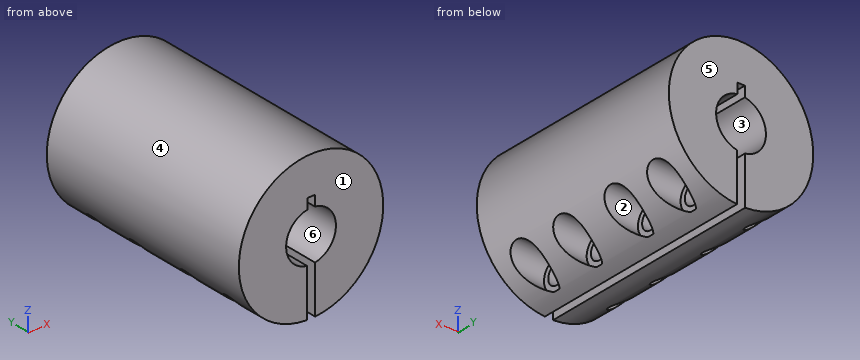
```python
from build123d import *

# Parameters (mm, degrees)
SKETCH1_R           = 14.5
SKETCH1_R_2         = 5
BOSS_EXTRUDE1_DEPTH = 22.5
CUT_EXTRUDE1_START  = -45
CUT_EXTRUDE1_DEPTH  = 45
SKETCH3_R           = 2
CUT_EXTRUDE2_DEPTH  = 40.465174521
SKETCH4_R           = 3
CUT_EXTRUDE3_DEPTH  = 10.5


with BuildPart() as part:
    # Sketch1 → Boss-Extrude1 (new, symmetric)
    with BuildSketch(Plane(origin=(0, 0, 0), x_dir=(1, 0, 0), z_dir=(0, 1, 0))):
        with Locations(Location((0, 0, 0), (0, 0, 90))):
            Circle(SKETCH1_R)
        with Locations(Location((0, 0, 0), (0, 0, 90))):
            Circle(SKETCH1_R_2, mode=Mode.SUBTRACT)
    extrude(amount=BOSS_EXTRUDE1_DEPTH, both=True)

    # Sketch2 → Cut-Extrude1 (cut)
    with BuildSketch(Plane.XZ.offset(22.5).offset(CUT_EXTRUDE1_START)):
        with BuildLine():
            Line((-0.824967477, -14.476513001), (-0.75, 7))
            Line((-0.75, 7), (0.75, 7))
            Line((0.75, 7), (0.824967477, -14.476513001))
            ThreePointArc((0.824967477, -14.476513001), (0, -14.5), (-0.824967477, -14.476513001))
        make_face()
    extrude(amount=CUT_EXTRUDE1_DEPTH, mode=Mode.SUBTRACT)

    # Sketch3 → Cut-Extrude2 (cut, through all)
    with BuildSketch(Plane(origin=(14.5, 0, 0), x_dir=(0, 0, -1), z_dir=(1, 0, 0))):
        with Locations((11, 16)):
            Circle(SKETCH3_R)
        with Locations((11, 6)):
            Circle(SKETCH3_R)
        with Locations((11, -6)):
            Circle(SKETCH3_R)
        with Locations((11, -16)):
            Circle(SKETCH3_R)
    extrude(amount=-CUT_EXTRUDE2_DEPTH, mode=Mode.SUBTRACT)

    # Sketch4 → Cut-Extrude3 (cut)
    with BuildSketch(Plane(origin=(14.5, 0, 0), x_dir=(0, 0, -1), z_dir=(1, 0, 0))):
        with Locations((11, 16)):
            Circle(SKETCH4_R)
        with Locations((11, 6)):
            Circle(SKETCH4_R)
        with Locations((11, -6)):
            Circle(SKETCH4_R)
        with Locations((11, -16)):
            Circle(SKETCH4_R)
    extrude(amount=-CUT_EXTRUDE3_DEPTH, mode=Mode.SUBTRACT)


solid = part.part
```
The listing builds one solid part. Answer for the finished solid, in the listing's coordinates (mm). Face numbers are marked on the shaded views. A direction names the side the tool comes from. Coordinates: 2 decimals unless noted, no trailing zeros. Loops run counter-clockwise (first coordinate to the right, second up) from the corner with the lowest first, then second, coordinate; pieces in that order, holes last. Notation, with made-up numbers: (31.25, 85) - (81.25, 85) arc R30 cw to (81.25, 121) - close; hole circle Ø4 at (1.25, 27). An arc over 180 degrees is marked (long way). Use a Markdown table: item, result. Add a question column.
1) The part is cut by section C-C, the plane y = 6. Give the vertices of the cut face in (x, z), and give its area (3 significant figures).
2) For the marked faces 1, 2 and 3, determine the directions among +Z, -Z, +X, -X, +Y, -Y from which every point of the face is accessible in a straight line to the end or side of a thin tool.
3) The part is cut by section A-A, the plane z = 0. Give the vertices of the cut face in (x, y), and give its area (3 significant figures).
4) The part is cut by section D-D, the plane z = 3. Give the vertices of the cut face in (x, y), and give its area (3 significant figures).
5) The mould has two halves that part along Z. Classify the marked faces 4, 5 and 6: released by +Z, released by -Z, zero draft, split by the parting line, or undercut.
6) The part is cut by section B-B, the plane x = 2.75. Give the vertices of the cut face in (y, z).
7) Find the intervals of material crossed by line 1 (Y direction, x = -8, z = -11); line 2 (Y direction, x = 9.25, z = -11); line 3 (Z direction, x = 2.75, y = 16), in increasing order.
8) Given pin 1 (6.5 mm diameter, centred on y = 6, z = -11, fed in from -X); pin 2 (0.8 mm diameter, centred on x = 0, y = -6.5, fed in from -Z); pin 3 (3.5 mm diameter, centred on y = -16, z = -11, fed in from +X); pin 4 (1.8 mm diameter, centred on y = 5, z = -12, fed in from +X), each flat-ended and moving along its own axis, determine where each tip first touches the part or whether it passes through.
Here are the results:
| question | item | result |
|---|---|---|
| 1 | outline | (-11.37, -9) - (-0.81, -9) - (-0.79, -4.94) arc R5 cw to (-0.76, 4.94) - (-0.75, 7) - (0.75, 7) - (0.76, 4.94) arc R5 cw to (0.79, -4.94) - (0.81, -9) - (4, -9) - (4, -8) - (12.09, -8) arc R14.5 ccw (long way) to start; (-6.42, -13) arc R14.5 ccw to (-0.82, -14.48) - (-0.82, -13) - close; (0.82, -14.48) arc R14.5 ccw to (4, -13.94) - (4, -13) - (0.82, -13) - close |
| 1 | area | 487 mm^2 |
| 2 | face 1 | +Z, -Z, +X, -X, -Y |
| 2 | face 2 | +X |
| 2 | face 3 | +Y, -Y |
| 3 | outline | (-14.5, -22.5) - (-5, -22.5) - (-5, 22.5) - (-14.5, 22.5) - close; (5, -22.5) - (14.5, -22.5) - (14.5, 22.5) - (5, 22.5) - close |
| 3 | area | 855 mm^2 |
| 4 | outline | (-14.19, -22.5) - (-4, -22.5) - (-4, 22.5) - (-14.19, 22.5) - close; (4, -22.5) - (14.19, -22.5) - (14.19, 22.5) - (4, 22.5) - close |
| 4 | area | 917 mm^2 |
| 5 | face 4 | split by the parting line |
| 5 | face 5 | zero draft |
| 5 | face 6 | undercut |
| 6 | outline | (-22.5, -14.24) - (22.5, -14.24) - (22.5, -4.18) - (-22.5, -4.18) - close; (-22.5, 4.18) - (22.5, 4.18) - (22.5, 14.24) - (-22.5, 14.24) - close; hole circle Ø4 at (-16, -11); hole circle Ø4 at (-6, -11); hole circle Ø4 at (6, -11); hole circle Ø4 at (16, -11) |
| 7 | line 1 | y = -22.5 to -18, -14 to -8, -4 to 4, 8 to 14, 18 to 22.5 |
| 7 | line 2 | y = -22.5 to -19, -13 to -9, -3 to 3, 9 to 13, 19 to 22.5 |
| 7 | line 3 | z = -14.24 to -13, -9 to -4.18, 4.18 to 14.24 |
| 8 | pin 1 | stops at x = -12.26 |
| 8 | pin 2 | stops at z = 7 |
| 8 | pin 3 | passes through |
| 8 | pin 4 | stops at x = 4 |
